Answer from the drawing. Dimensions are ordinates in mm from the lowest x, y and z of the part. A direction names the side the tool comes from. Give positions to 0.01 mm unless a question says otherwise; leave off trailing zeros. Loops run counter-clockwise (first coordinate to the right, second up) from the corner with the lowest first, then second, coordinate; pieces in that order, holes last. Notation, with made-up numbers: (43, 68.25) -> (89, 68.25) arc R27 cw to (89, 91.25) -> close; hole circle Ø3 at (87, 24.25). An arc over 180 degrees is marked (long way). Write each question's results on one line, items separated by ' | '. Start each with the question number.
Item 1: Section B-B on z = 15.25 is taken. Write down the section's boundary in (x, y), and give its area (3 significant figures).
Item 2: Which of the six approach directions +Z, -Z, +X, -X, +Y, -Y give full straight-line access (tool end or side, diameter ignored) to the marked faces 1 and 2?
Item 3: Each of these flat-tipped pins is pushed along its axis until it touches: P1, Ø10, axis at x = 7.5, z = 17.5, coming from the +Y side; P2, Ø6, axis at x = 10, z = 7, coming from the +Y side; P3, Ø4, axis at x = 5.5, y = 40, coming from the -Z side. Where does it stop, or does it pass through?
Item 4: Section D-D on z = 10 is taken. Write down the section's boundary in (x, y), and give its area (4 significant figures).
Item 5: Section A-A on x = 10 is taken. Write down the section's boundary in (y, z), and give its area (4 significant figures).
Item 6: Find the intervals of material crossed by line 1 (Y direction, x = 7.5, z = 3); line 2 (Y direction, x = 19, z = 18); line 3 (X direction, y = 36.5, z = 9), in increasing order.
Item 7: Section C-C on y = 37.5 is taken. Write down the section's boundary in (x, z), and give its area (3 significant figures).
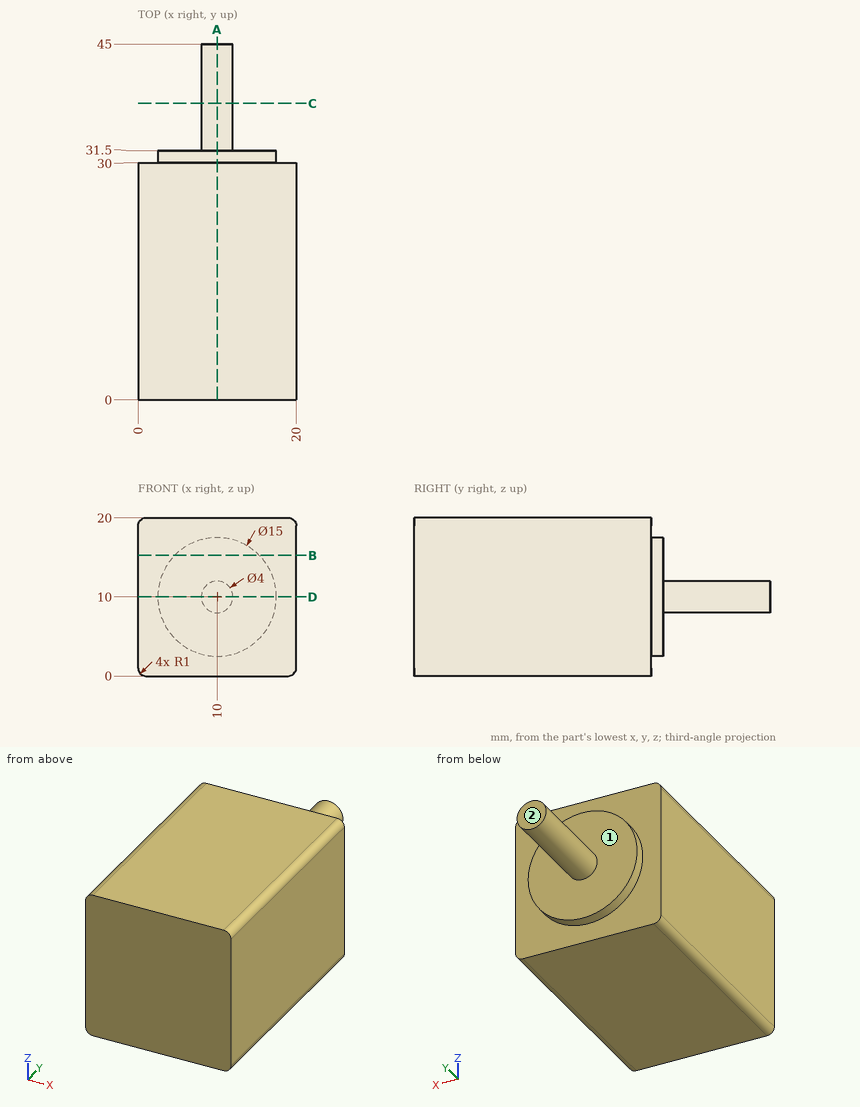
Findings:
1) outline: (0, 0) -> (20, 0) -> (20, 30) -> (15.36, 30) -> (15.36, 31.5) -> (4.64, 31.5) -> (4.64, 30) -> (0, 30) -> close | area: 616 mm2
2) face 1: +Y | face 2: +Z, -Z, +X, -X, +Y
3) P1: y = 31.5 | P2: y = 45 | P3: through
4) outline: (0, 0) -> (20, 0) -> (20, 30) -> (17.5, 30) -> (17.5, 31.5) -> (12, 31.5) -> (12, 45) -> (8, 45) -> (8, 31.5) -> (2.5, 31.5) -> (2.5, 30) -> (0, 30) -> close | area: 676.5 mm2
5) outline: (0, 0) -> (30, 0) -> (30, 2.5) -> (31.5, 2.5) -> (31.5, 8) -> (45, 8) -> (45, 12) -> (31.5, 12) -> (31.5, 17.5) -> (30, 17.5) -> (30, 20) -> (0, 20) -> close | area: 676.5 mm2
6) line 1: 0 to 31.5 | line 2: 0 to 30 | line 3: 8.27 to 11.73
7) outline: circle Ø4 at (10, 10) | area: 12.6 mm2
